Geometry check sheet. Reference: the model listing, model coordinates, mm. A direction names the side the tool comes from. Round coordinates to 2 decimals unless told otherwise and drop trailing zeros. Write each loop counter-clockwise with the first axis right and the second up, starting at its lowest first coordinate (ties: lowest second). Pieces come first, ordered by that corner, then holes. Notation, with made-up numbers: M 23.25,43 L 42.25,43 A26 cw 42.25,61 Z; hole C -29.75,-3.5 d2. An arc over 180 degrees is marked long. Put each result on its own line as item: value. Start each with the question number.
(1) Tool access check on faces 1 (the flat face through (25, -7, 5)), 2 (the flat face through (45, 0, 5)), 3 (the flat face through (45, -7, 0)). Record the directions out of +Z, -Z, +X, -X, +Y, -Y that give a thin tool (end or side, any length) a straight path to the whole face; none if there is none.
(2) Section check C-C on y = -8. Record the cut outline in (x, z).
(3) Section check D-D on y = -15.25. Record the cut outline in (x, z), then the cut area to 3 significant figures.
(4) Section check A-A on z = 4.5. Record the cut outline in (x, y), then the cut area to 3 significant figures.
(5) Section check B-B on x = 39. Record the cut outline in (y, z).
(6) Gauge pin test, flat ends, axial feed: pin 1 (8 mm diameter, centred on x = 6.5, y = -8, fed in from -Z); pin 2 (3 mm diameter, centred on y = -5, z = -2, fed in from -X); pin 3 (6.5 mm diameter, centred on y = -4.5, z = -3.5, fed in from +X); pin 4 (1 mm diameter, centred on x = 25, z = -1.5, fed in from +Y). Record the tip position at first contact, or that the pin passes through.
(7) Material ranges on probe 1 along X at (y, z) = (-12, 5.75); probe 2 along Y at (x, z) = (16.75, 4.5); probe 3 along Y at (x, z) = (4.5, 4.5), recorded low to high.
(8) Mould release check, pull along X, two halves, no side actions. Record for faces 4 (the flat face through (20, -2, 0)), 5 (the flat face through (0, -8, 4)), 6 (the flat face through (37.036, -1.115, -2.727)): pulls with the +X half, pulls with the -X half, needs draft (parallel to the pull), parting line crosses it, or undercut.
from build123d import *

# Parameters (mm, degrees)
BOSS_EXTRUDE1_DEPTH = 9
SKETCH2_R           = 2.5
CUT_EXTRUDE1_DEPTH  = 56
SKETCH5_W           = 5
SKETCH5_H           = 7
BOSS_EXTRUDE2_DEPTH = 6
CUT_EXTRUDE3_DEPTH  = 30
CUT_EXTRUDE4_DEPTH  = 60


with BuildPart() as part:
    # Sketch1 → Boss-Extrude1 (new body)
    with BuildSketch(Plane.XY):
        Polygon((0, 0), (10.5, 0), (10.5, 11), (39.5, 11), (39.5, 0), (50, 0), (50, -19), (40, -19), (40, -7), (10, -7), (10, -19), (0, -19), align=None)
    extrude(amount=BOSS_EXTRUDE1_DEPTH)

    # Sketch2 → Cut-Extrude1 (cut)
    with BuildSketch(Plane.ZY):
        with Locations((4.5, -14.5)):
            Circle(SKETCH2_R)
        with Locations((4.5, 6.5)):
            Circle(SKETCH2_R)
    extrude(amount=-CUT_EXTRUDE1_DEPTH, mode=Mode.SUBTRACT)

    # Sketch5 → Boss-Extrude2 (add)
    with BuildSketch(Plane(origin=(0, 0, 0), x_dir=(-1, 0, 0), z_dir=(0, 0, -1))):
        with Locations((-13.001, -3.5)):
            Rectangle(SKETCH5_W, SKETCH5_H)
        with Locations((-37.001, -3.5)):
            Rectangle(SKETCH5_W, SKETCH5_H)
    extrude(amount=BOSS_EXTRUDE2_DEPTH)

    # Sketch6 → Cut-Extrude3 (cut)
    with BuildSketch(Plane(origin=(39.501, 0, 0), x_dir=(0, 0, -1), z_dir=(1, 0, 0))):
        with BuildLine():
            Line((0, -7), (5.378584213, -4.8))
            ThreePointArc((5.378584213, -4.8), (5.830236175, -4.431844931), (6, -3.87443315))
            Line((6, -3.87443315), (6, -3.12556685))
            ThreePointArc((6, -3.12556685), (5.830236175, -2.568155069), (5.378584213, -2.2))
            Line((5.378584213, -2.2), (0, 0))
            Line((0, 0), (0, 0.711055657))
            Line((0, 0.711055657), (7.382706711, 0.711055657))
            Line((7.382706711, 0.711055657), (7.382706711, -8.433389186))
            Line((7.382706711, -8.433389186), (0, -8.433389186))
            Line((0, -8.433389186), (0, -7))
        make_face()
    extrude(amount=-CUT_EXTRUDE3_DEPTH, mode=Mode.SUBTRACT)

    # Sketch7 → Cut-Extrude4 (cut)
    with BuildSketch(Plane(origin=(50, 0, 0), x_dir=(0, 0, -1), z_dir=(1, 0, 0))):
        with BuildLine():
            Line((0, 6.5), (1.728310858, 6.5))
            Line((1.728310858, 6.5), (1.728310858, 12.31373859))
            Line((1.728310858, 12.31373859), (-10.493151676, 12.31373859))
            Line((-10.493151676, 12.31373859), (-10.493151676, 4.742580982))
            Line((-10.493151676, 4.742580982), (-9, 6.5))
            ThreePointArc((-9, 6.5), (-4.5, 11), (0, 6.5))
        make_face()
        with BuildLine():
            Line((0, -14.5), (1.22869132, -14.5))
            Line((1.22869132, -14.5), (1.22869132, -21.122338154))
            Line((1.22869132, -21.122338154), (-10.493151676, -21.122338154))
            Line((-10.493151676, -21.122338154), (-10.493151676, -14.5))
            Line((-10.493151676, -14.5), (-9, -14.5))
            ThreePointArc((-9, -14.5), (-4.5, -19), (0, -14.5))
        make_face()
    extrude(amount=-CUT_EXTRUDE4_DEPTH, mode=Mode.SUBTRACT)


solid = part.part
Answers follow:
1. face 1: +Z, -Z, -Y
1. face 2: +Z, -Z, +X, +Y
1. face 3: -Z, +X, +Y, -Y
2. outline: M 0,0 L 10,0 L 10,9 L 0,9 Z; M 40,0 L 50,0 L 50,9 L 40,9 Z
3. outline: M 0,0.06 L 10,0.06 L 10,2.12 L 0,2.12 Z; M 0,6.88 L 10,6.88 L 10,8.94 L 0,8.94 Z; M 40,0.06 L 50,0.06 L 50,2.12 L 40,2.12 Z; M 40,6.88 L 50,6.88 L 50,8.94 L 40,8.94 Z
3. area: 82.1 mm^2
4. outline: M 0,-19 L 10,-19 L 10,-17 L 0,-17 Z; M 0,-12 L 10,-12 L 10,-7 L 40,-7 L 40,-12 L 50,-12 L 50,0 L 39.5,0 L 39.5,4 L 10.5,4 L 10.5,0 L 0,0 Z; M 10.5,9 L 39.5,9 L 39.5,11 L 10.5,11 Z; M 40,-19 L 50,-19 L 50,-17 L 40,-17 Z
4. area: 664 mm^2
5. outline: M -7,0 L -4.8,-5.38 A1 ccw -3.87,-6 L -3.13,-6 A1 ccw -2.2,-5.38 L 0,0 L 6.5,0 A4.5 ccw 6.5,9 L -7,9 Z; hole C 6.5,4.5 d5
6. pin 1: stops at z = 0
6. pin 2: stops at x = 10.5
6. pin 3: stops at x = 39.5
6. pin 4: passes through
7. probe 1: x = 0 to 10, 40 to 50
7. probe 2: y = -7 to 4, 9 to 11
7. probe 3: y = -19 to -17, -12 to 0
8. face 4: undercut
8. face 5: pulls with the -X half
8. face 6: needs draft
